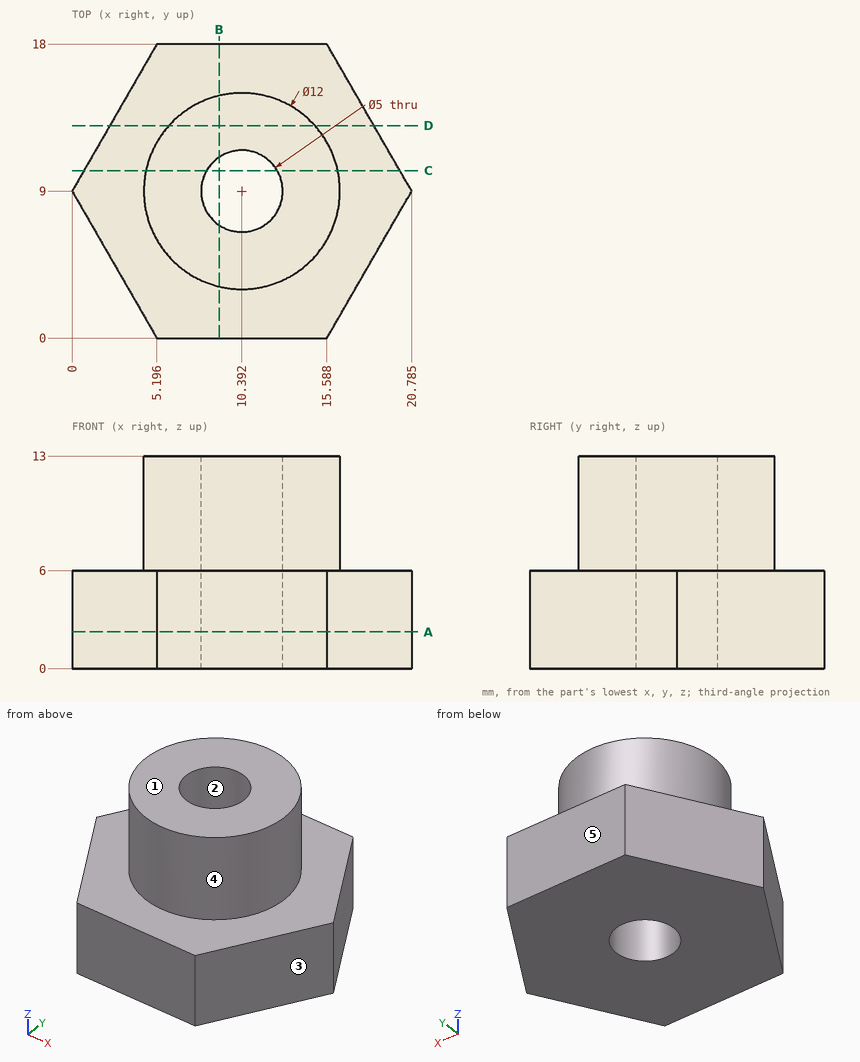
The drawing under review shows one solid part. Ordinate dimensions are in mm from its lowest x, y, z. A direction names the side the tool comes from. Coordinates: 2 decimals unless noted, no trailing zeros. Loops run counter-clockwise (first coordinate to the right, second up) from the corner with the lowest first, then second, coordinate; pieces in that order, holes last. Notation, with made-up numbers: M 78,26 L 130,26 A24 cw 130,57 Z; hole C 47,35.5 d5. An arc over 180 degrees is marked long. Use one line per item in the form item = value.
(1) Consider section A-A (z = 2.25). Write out the cut boundary in (x, y) (1 decimal).
Return value:
outline = M 0,9 L 5.2,0 L 15.6,0 L 20.8,9 L 15.6,18 L 5.2,18 Z; hole C 10.4,9 d5
(2) Consider section B-B (x = 9). Write out the cut boundary in (y, z).
Return value:
outline = M 0,0 L 6.92,0 L 6.92,13 L 3.16,13 L 3.16,6 L 0,6 Z; M 11.08,0 L 18,0 L 18,6 L 14.84,6 L 14.84,13 L 11.08,13 Z
(3) For the marked faces 4 and 5, list the 3-axis set-ups (+Z, -Z, +X, -X, +Y, -Y) from which the entire face can be reached by the end or side of a thin tool; tool diameter is ignored.
Return value:
face_4 = +Z
face_5 = +Z, -Z, +X, -X, +Y
(4) Draft analysis for pull direction Y (two halves, no side actions). For the marked faces 1, 2 and 3, state which applies: pulls with the +Y half, pulls with the -Y half, needs draft (parallel to the pull), parting line crosses it, or undercut.
Return value:
face_1 = needs draft
face_2 = undercut
face_3 = pulls with the -Y half
(5) Consider section C-C (y = 10.25). Write out the cut boundary in (x, z).
Return value:
outline = M 0.72,0 L 8.23,0 L 8.23,13 L 4.52,13 L 4.52,6 L 0.72,6 Z; M 12.56,0 L 20.06,0 L 20.06,6 L 16.26,6 L 16.26,13 L 12.56,13 Z
(6) For line 1 along Y through (x, z) = (10.5, 7); line 2 along Z through (x, y) = (5.75, 16.5); line 3 along X through (y, z) = (8.5, 5.5) (1 decimal), list the stretches that pass through material, from the lowest coordinate up. Write a range as from..to.
Return value:
line_1 = 3..6.5, 11.5..15
line_2 = 0..6
line_3 = 0.3..7.9, 12.8..20.5
(7) Consider section D-D (y = 13). Write out the cut boundary in (x, z) (1 decimal), and give its area (3 significant figures).
Return value:
outline = M 2.3,0 L 18.5,0 L 18.5,6 L 14.9,6 L 14.9,13 L 5.9,13 L 5.9,6 L 2.3,6 Z
area = 160 mm2
(8) Clearance check with flat-ended pins moving along their axes: P1, Ø1.5, axis at y = 10, z = 2.5, coming from the +X side; P2, Ø2, axis at x = 17.5, z = 6, coming from the +Y side; P3, Ø2, axis at x = 2.5, y = 2.5, coming from the -Z side. State where each tip first meets the part, or that it passes through.
Return value:
P1 = 20.64
P2 = 16.42
P3 = through
